```python
from build123d import *

# Parameters (mm, degrees)
SKETCH3_W              = 83
SKETCH3_H              = 83
BODY_DEPTH             = 15
SHELL_T                = -3
SKETCH4_W              = 6
SKETCH4_H              = 6
SKETCH4_R              = 1.85
INSERTS_SUPPPORT_DEPTH = 25
CHAMFER1_SIZE          = 3
CHAMFER2_SIZE          = 1
SKETCH5_R              = 1.25
AIR_EXTRACTION_DEPTH   = 95.001329778
CHAMFER3_SIZE          = 1.25
SKETCH7_R              = 3.85
SKETCH7_R_2            = 1.85
BOSS_EXTRUDE1_DEPTH    = 4


with BuildPart() as part:
    # Sketch3 → Body (new, symmetric)
    with BuildSketch(Plane(origin=(0, 0, 0), x_dir=(1, 0, 0), z_dir=(0, 1, 0))):
        Rectangle(SKETCH3_W, SKETCH3_H)
    extrude(amount=BODY_DEPTH, both=True)

    # Shell
    shell_openings = [part.faces().sort_by_distance(p)[0] for p in [
        (0, 15, 0),
    ]]
    offset(amount=SHELL_T, openings=shell_openings, kind=Kind.INTERSECTION)

    # Sketch4 → Inserts_Suppport (add)
    # profile 1 of 4: a face of its own
    with BuildSketch(Plane(origin=(0, -12, 0), x_dir=(1, 0, 0), z_dir=(0, 1, 0))):
        with Locations((-35.5, 35.5)):
            Rectangle(SKETCH4_W, SKETCH4_H)
        with Locations(Location((-35.5, 35.5, 0), (0, 0, 270))):
            Circle(SKETCH4_R, mode=Mode.SUBTRACT)
    # profile 2 of 4: a face of its own
    with BuildSketch(Plane(origin=(0, -12, 0), x_dir=(1, 0, 0), z_dir=(0, 1, 0))):
        with Locations((35.5, 35.5)):
            Rectangle(SKETCH4_W, SKETCH4_H)
        with Locations(Location((35.5, 35.5, 0), (0, 0, 270))):
            Circle(SKETCH4_R, mode=Mode.SUBTRACT)
    # profile 3 of 4: a face of its own
    with BuildSketch(Plane(origin=(0, -12, 0), x_dir=(1, 0, 0), z_dir=(0, 1, 0))):
        with Locations((35.5, -35.5)):
            Rectangle(SKETCH4_W, SKETCH4_H)
        with Locations(Location((35.5, -35.5, 0), (0, 0, 270))):
            Circle(SKETCH4_R, mode=Mode.SUBTRACT)
    # profile 4 of 4: a face of its own
    with BuildSketch(Plane(origin=(0, -12, 0), x_dir=(1, 0, 0), z_dir=(0, 1, 0))):
        with Locations((-35.5, -35.5)):
            Rectangle(SKETCH4_W, SKETCH4_H)
        with Locations(Location((-35.5, -35.5, 0), (0, 0, 270))):
            Circle(SKETCH4_R, mode=Mode.SUBTRACT)
    extrude(amount=INSERTS_SUPPPORT_DEPTH)

    # Chamfer1
    chamfer1_edges = [part.edges().sort_by_distance(p)[0] for p in [
        (-41.5, 0, -41.5),
        (41.5, 0, -41.5),
        (41.5, 0, 41.5),
        (-41.5, 0, 41.5),
    ]]
    chamfer(chamfer1_edges, length=CHAMFER1_SIZE)

    # Chamfer2
    chamfer2_edges = [part.edges().sort_by_distance(p)[0] for p in [
        (0, 15, 41.5),
        (-41.5, 15, 0),
        (41.5, 15, 0),
        (0, 15, -41.5),
    ]]
    chamfer(chamfer2_edges, length=CHAMFER2_SIZE)

    # Sketch5 → Air_Extraction (cut, through all)
    with BuildSketch(Plane.XY.offset(41.5)):
        with Locations((-7.5, 7.5)):
            Circle(SKETCH5_R)
        with Locations((-7.5, -7.5)):
            Circle(SKETCH5_R)
        with Locations((7.5, -7.5)):
            Circle(SKETCH5_R)
        with Locations((7.5, 7.5)):
            Circle(SKETCH5_R)
        with BuildLine():
            Line((-4.5, 3.75), (-4.5, -3.75))
            ThreePointArc((-4.5, -3.75), (-5.5, -4.75), (-6.5, -3.75))
            Line((-6.5, -3.75), (-6.5, 3.75))
            ThreePointArc((-6.5, 3.75), (-5.5, 4.75), (-4.5, 3.75))
        make_face()
        with BuildLine():
            Line((-0.833333333, 3.75), (-0.833333333, -3.75))
            ThreePointArc((-0.833333333, -3.75), (-1.833333333, -4.75), (-2.833333333, -3.75))
            Line((-2.833333333, -3.75), (-2.833333333, 3.75))
            ThreePointArc((-2.833333333, 3.75), (-1.833333333, 4.75), (-0.833333333, 3.75))
        make_face()
        with BuildLine():
            Line((2.833333333, 3.75), (2.833333333, -3.75))
            ThreePointArc((2.833333333, -3.75), (1.833333333, -4.75), (0.833333333, -3.75))
            Line((0.833333333, -3.75), (0.833333333, 3.75))
            ThreePointArc((0.833333333, 3.75), (1.833333333, 4.75), (2.833333333, 3.75))
        make_face()
        with BuildLine():
            Line((6.5, 3.75), (6.5, -3.75))
            ThreePointArc((6.5, -3.75), (5.5, -4.75), (4.5, -3.75))
            Line((4.5, -3.75), (4.5, 3.75))
            ThreePointArc((4.5, 3.75), (5.5, 4.75), (6.5, 3.75))
        make_face()
    extrude(amount=-AIR_EXTRACTION_DEPTH, mode=Mode.SUBTRACT)

    # Chamfer3
    chamfer3_edges = [part.edges().sort_by_distance(p)[0] for p in [
        (6.25, 7.5, -41.5),
        (6.25, 7.5, 41.5),
        (6.25, -7.5, -41.5),
        (6.25, -7.5, 41.5),
        (-8.75, 7.5, -41.5),
        (-8.75, 7.5, 41.5),
        (-8.75, -7.5, -41.5),
        (-8.75, -7.5, 41.5),
    ]]
    chamfer(chamfer3_edges, length=CHAMFER3_SIZE)

    # Sketch7 → Boss-Extrude1 (add)
    # profile 1 of 4: a face of its own
    with BuildSketch(Plane(origin=(0, -12, 0), x_dir=(1, 0, 0), z_dir=(0, 1, 0))):
        with Locations(Location((7, 27.5, 0), (0, 0, 270))):
            Circle(SKETCH7_R)
        with Locations(Location((7, 27.5, 0), (0, 0, 270))):
            Circle(SKETCH7_R_2, mode=Mode.SUBTRACT)
    # profile 2 of 4: a face of its own
    with BuildSketch(Plane(origin=(0, -12, 0), x_dir=(1, 0, 0), z_dir=(0, 1, 0))):
        with Locations(Location((-33, 27.5, 0), (0, 0, 270))):
            Circle(SKETCH7_R)
        with Locations(Location((-33, 27.5, 0), (0, 0, 270))):
            Circle(SKETCH7_R_2, mode=Mode.SUBTRACT)
    # profile 3 of 4: a face of its own
    with BuildSketch(Plane(origin=(0, -12, 0), x_dir=(1, 0, 0), z_dir=(0, 1, 0))):
        with Locations(Location((-33, -27.5, 0), (0, 0, 270))):
            Circle(SKETCH7_R)
        with Locations(Location((-33, -27.5, 0), (0, 0, 270))):
            Circle(SKETCH7_R_2, mode=Mode.SUBTRACT)
    # profile 4 of 4: a face of its own
    with BuildSketch(Plane(origin=(0, -12, 0), x_dir=(1, 0, 0), z_dir=(0, 1, 0))):
        with Locations(Location((7, -27.5, 0), (0, 0, 270))):
            Circle(SKETCH7_R)
        with Locations(Location((7, -27.5, 0), (0, 0, 270))):
            Circle(SKETCH7_R_2, mode=Mode.SUBTRACT)
    extrude(amount=BOSS_EXTRUDE1_DEPTH)


solid = part.part
```
For this review, take the finished solid that the model builds, in its own axes (mm). A direction names the side the tool comes from. Round coordinates to 2 decimals unless told otherwise and drop trailing zeros. Write each loop counter-clockwise with the first axis right and the second up, starting at its lowest first coordinate (ties: lowest second). Pieces come first, ordered by that corner, then holes.
1) Insertion check: pin 1 Ø4 at (x, y) = (-7.5, -7.5) entering from -Z; pin 2 Ø1.5 at (x, z) = (13, 5) entering from +Y; pin 3 Ø3.5 at (y, z) = (0.5, -40.5) entering from +X. Each pin has a flat end and moves straight along its axis. Give the tip position at first contact, or say it passes through.
Answer below:
pin 1: stops at z = -41
pin 2: stops at y = -12
pin 3: stops at x = 41.25
2) Mouldability with a two-part tool opening along Y and no side actions: class faces 6 (the face through (6.25, 7.55, 39.39)), 7 (the face through (-2.833, 0, -40)), 8 (the face through (-33, -12, -28)), 9 (the face through (40, 0, 40)) as +Y half, -Y half, draft (parallel to the pull), parting line (faces both ways), or undercut.
Answer below:
face 6: undercut
face 7: undercut
face 8: +Y half
face 9: draft
3) Take a section at A-A on y = -11. State how many separate pieces and enclosed holes the cut face has, then the cut area to 3 significant figures.
Answer below:
separate pieces: 5
enclosed holes: 9
area: 1,190 mm2
4) Take a section at B-B on x = 35.5. Give the boundary of the cut face in (y, z), then the cut area to 3 significant figures.
Answer below:
outline: (-15, -41.5) - (14, -41.5) - (15, -40.5) - (15, -38.5) - (13, -38.5) - (13, -37.35) - (-12, -37.35) - (-12, -33.65) - (13, -33.65) - (13, -32.5) - (-12, -32.5) - (-12, 32.5) - (13, 32.5) - (13, 33.65) - (-12, 33.65) - (-12, 37.35) - (13, 37.35) - (13, 38.5) - (15, 38.5) - (15, 40.5) - (14, 41.5) - (-15, 41.5) - close
area: 525 mm2
5) Take a section at D-D on z = 27.5. Give the boundary of the cut face in (x, y).
Answer below:
outline: (-41.5, -15) - (41.5, -15) - (41.5, 14) - (40.5, 15) - (38.5, 15) - (38.5, -12) - (10.85, -12) - (10.85, -8) - (8.85, -8) - (8.85, -12) - (5.15, -12) - (5.15, -8) - (3.15, -8) - (3.15, -12) - (-29.15, -12) - (-29.15, -8) - (-31.15, -8) - (-31.15, -12) - (-34.85, -12) - (-34.85, -8) - (-36.85, -8) - (-36.85, -12) - (-38.5, -12) - (-38.5, 15) - (-40.5, 15) - (-41.5, 14) - close
6) Machinability: for faces 1 (the face through (6.25, -7.45, -39.36)), 2 (the face through (6.25, -7.45, 39.39)), 3 (the face through (-1, -15, -1)), 4 (the face through (0.833, 0, -40)), 5 (the face through (7.169, -10.028, 23.654)), which of the approach directions +Z, -Z, +X, -X, +Y, -Y give a long, thin tool a straight path to every point of the face, cutting with its end or side? Answer none if there is none.
Answer below:
face 1: -Z
face 2: +Z
face 3: +Z, -Z, +X, -X, -Y
face 4: +Z, -Z
face 5: +Y
7) For line 1 along Y through (x, z) = (7.5, 39.55); line 2 along X through (y, z) = (7.5, 30.5), list the stretches that pass through material, from the lowest coordinate up.
Answer below:
line 1: y = -15 to -8.75, -6.25 to 6.25, 8.75 to 15
line 2: x = -41.5 to -38.5, 38.5 to 41.5
